```python
from build123d import *

# Parameters (mm, degrees)
F1_DEPTH = 8.95
F2_W     = 50
F2_H     = 28
F2_W_2   = 34.5
F2_H_2   = 17.9
F3_DEPTH = 6
F5_DEPTH = 4.55
F6_R     = 3.5
F7_R     = 9


with BuildPart() as f1:
    # F0 (on Front) → F1 (new body, symmetric)
    with BuildSketch(Plane.XZ):
        Polygon((20.541627, 50.516934), (-13.958373, 50.516934), (15.516038, -59.483066), (50.016038, -59.483066), align=None)
    extrude(amount=F1_DEPTH, both=True)

    # F2 (on face) → F3 (join)
    with BuildSketch(Plane(origin=(0, 0, -59.483066), x_dir=(1, 0, 0), z_dir=(0, 0, -1))):
        with Locations((32.766038, 0)):
            Rectangle(F2_W, F2_H)
        with Locations((32.766038, 0)):
            Rectangle(F2_W_2, F2_H_2, mode=Mode.SUBTRACT)
        with Locations((32.766038, 0)):
            Rectangle(F2_W_2, F2_H_2)
    extrude(amount=F3_DEPTH)

    # F4 (on Front) → F5 (cut, symmetric)
    with BuildSketch(Plane.XZ):
        Polygon((12.841627, 50.516934), (-6.258373, 50.516934), (20.536546, -49.483066), (39.636546, -49.483066), align=None)
    extrude(amount=F5_DEPTH, both=True, mode=Mode.SUBTRACT)

    # F6
    f6_edges = [f1.edges().sort_by_distance(p)[0] for p in [
        (57.766038, -14, -62.483066),
        (57.766038, 14, -62.483066),
    ]]
    fillet(f6_edges, radius=F6_R)

    # F7
    f7_edges = [f1.edges().sort_by_distance(p)[0] for p in [
        (7.766038, -14, -62.483066),
        (7.766038, 14, -62.483066),
    ]]
    fillet(f7_edges, radius=F7_R)


solid = f1.part
```
Read the model definition and answer for the solid it produces. Units are mm, in the model's axes. A direction names the side the tool comes from. Give positions to 0.01 mm unless a question says otherwise; leave off trailing zeros. Write each loop counter-clockwise with the first axis right and the second up, starting at its lowest first coordinate (ties: lowest second). Pieces come first, ordered by that corner, then holes. Notation, with made-up numbers: (35.25, -39.5) - (60.25, -39.5) arc R28 cw to (60.25, -6.5) - close; hole circle Ø6 at (78, -32). An arc over 180 degrees is marked (long way). Write item = value, one per line. Start each with the question number.
Item 1: A tool of negligible diameter and unlimited length cuts with its end or side. For faces 4 (the cylindrical face through (10.33, -11.29, -62.53)), 5 (the flat face through (26.427, -0.064, -0.183)), 6 (the cylindrical face through (10.47, 11.43, -62.53)), from which of +Z, -Z, +X, -X, +Y, -Y can it reach the whole face along a straight path? Write none if from no direction.
Item 2: Find section A-A (y = -2). Give the vertices of the cut face in (x, z).
Item 3: Find section D-D (x = 48). Give the vertices of the cut face in (y, z), then the cut area to 3 significant figures.
Item 4: The mould has two halves that part along Z. Classify faces 1 (the flat face through (57.766, 0, -62)), 2 (the flat face through (4, 6, 50.517)), 3 (the flat face through (0.57, -0.13, -3.71)): +Z half, -Z half, draft (parallel to the pull), parting line (faces both ways), or undercut.
Item 5: Each of these flat-tipped pins is pushed along its axis until it touches: P1, Ø12, axis at x = 11, z = 24, coming from the +Y side; P2, Ø6, axis at y = 2, z = -18, coming from the -X side; P3, Ø23, axis at x = 16.5, z = 15, coming from the -Y side. Where does it stop, or does it pass through?
Item 6: Find the intervals of material crossed by probe 1 along Y at (x, z) = (38, -49); probe 2 along Z at (x, y) = (26.5, -10.75); probe 3 along X at (y, z) = (1.75, 44.5), in increasing order. Write a range as [from, to].
Item 7: Find section C-C (x = 34). Give the vertices of the cut face in (y, z), then the cut area to 3 significant figures.
Item 8: Find section B-B (z = -31). Give the vertices of the cut face in (x, y), then the cut area to 3 significant figures.
Response:
q1.face_4 = -Z, -X, -Y
q1.face_5 = none
q1.face_6 = -Z, -X, +Y
q2.outline = (-13.96, 50.52) - (15.52, -59.48) - (7.77, -59.48) - (7.77, -65.48) - (57.77, -65.48) - (57.77, -59.48) - (50.02, -59.48) - (20.54, 50.52) - (12.84, 50.52) - (39.64, -49.48) - (20.54, -49.48) - (-6.26, 50.52) - close
q3.outline = (-14, -65.48) - (14, -65.48) - (14, -59.48) - (8.95, -59.48) - (8.95, -51.96) - (-8.95, -51.96) - (-8.95, -59.48) - (-14, -59.48) - close
q3.area = 303 mm²
q4.face_1 = draft
q4.face_2 = +Z half
q4.face_3 = undercut
q5.P1 = 8.95
q5.P2 = 3.6
q5.P3 = -8.95
q6.probe_1 = [-8.95, -4.55], [4.55, 8.95]
q6.probe_2 = [-65.48, -59.48]
q6.probe_3 = [-12.35, -4.65], [14.45, 22.15]
q7.outline = (-14, -65.48) - (14, -65.48) - (14, -59.48) - (8.95, -59.48) - (8.95, 0.29) - (-8.95, 0.29) - (-8.95, -59.48) - (-14, -59.48) - close; hole (-4.55, -49.48) - (4.55, -49.48) - (4.55, -28.45) - (-4.55, -28.45) - close
q7.area = 1,050 mm²
q8.outline = (7.88, -8.95) - (42.38, -8.95) - (42.38, 8.95) - (7.88, 8.95) - close; hole (15.58, -4.55) - (34.68, -4.55) - (34.68, 4.55) - (15.58, 4.55) - close
q8.area = 444 mm²
